Input: part model. Units: mm. Frame: model coordinates. A direction names the side the tool comes from. Round coordinates to 2 decimals unless told otherwise and drop trailing zeros. Loops run counter-clockwise (first coordinate to the right, second up) from the corner with the lowest first, then second, coordinate; pieces in that order, holes last.
(1) Cut plane C-C, the plane x = 0. Output: boundary loops of the cut face in (y, z) (1 decimal), and give its area (3 significant figures).
(2) Line query: line 1 (X direction, y = 328, z = 3); line 2 (X direction, y = 304.8, z = 1.85); line 3 (X direction, y = 330.2, z = 1.4). Output: solid intervals per line, ascending.
(3) Cut plane A-A, the plane x = -50.8. Output: boundary loops of the cut face in (y, z) (3 decimals).
(4) Draft query along Y for faces 3 (the face through (-12.7, 282, 2)), 4 (the face through (1.372, 281.552, 1.61)), 5 (the face through (-0.7, 246.15, 1.57)), 6 (the face through (-0.553, 327.708, 1.61)). Return one class per face: released by +Y, released by -Y, zero draft, split by the parting line, or undercut.
(5) Cut plane B-B, the plane z = 1.6. Output: boundary loops of the cut face in (x, y).
(6) Access query for faces 1 (the face through (-48, 317.5, 2)), 2 (the face through (-14, 316, 0)). Directions: +Z, -Z, +X, -X, +Y, -Y. A direction counts if a zero-diameter tool reaches every point of the face in a straight line with its end or side. Return the directions, or none.
(7) First-contact query: pin 1 Ø3 at (x, y) = (0, 254) entering from -Z; pin 2 Ø1.5 at (y, z) = (299.5, 1) entering from -X. Flat tips, straight axial feed; report the tip coordinate or a pass-through.
(8) Cut plane D-D, the plane y = 330.2. Output: boundary loops of the cut face in (x, z) (1 decimal).
from build123d import *

# Parameters (mm, degrees)
BOSS_EXTRUDE1_DEPTH        = 3.175
FILLET1_R                  = 6.35
F_10_CLEARANCE_HOLE1_D     = 5.1054
F_10_CLEARANCE_HOLE1_DEPTH = 9.906
F_10_CLEARANCE_HOLE1_TIP   = 1.533816902


with BuildPart() as part:
    # Sketch1 → Boss-Extrude1 (new body)
    with BuildSketch(Plane.XY):
        with BuildLine():
            Line((-12.7, 247.65), (-12.7, 317.5))
            Line((-12.7, 317.5), (-82.55, 317.5))
            Line((-82.55, 317.5), (-84.832797429, 335.762379435))
            ThreePointArc((-84.832797429, 335.762379435), (-83.292289329, 340.752446277), (-78.531832912, 342.9))
            Line((-78.531832912, 342.9), (6.35, 342.9))
            ThreePointArc((6.35, 342.9), (10.840128061, 341.040128061), (12.7, 336.55))
            Line((12.7, 336.55), (12.7, 251.668167088))
            ThreePointArc((12.7, 251.668167088), (10.552446277, 246.907710671), (5.562379435, 245.367202571))
            Line((5.562379435, 245.367202571), (-12.7, 247.65))
        make_face()
    extrude(amount=BOSS_EXTRUDE1_DEPTH)

    # Fillet1
    fillet1_edges = [part.edges().sort_by_distance(p)[0] for p in [
        (-12.7, 247.65, 1.5875),
        (-12.7, 317.5, 1.5875),
        (-82.55, 317.5, 1.5875),
    ]]
    fillet(fillet1_edges, radius=FILLET1_R)

    # #10 Clearance Hole1
    with Locations(Plane(origin=(0, 0, 0), x_dir=(-1, 0, 0), z_dir=(0, 0, -1))):
        with Locations((0, 330.2), (0, 304.8), (0, 279.4), (25.4, 330.2), (0, 254), (50.8, 330.2), (76.2, 330.2)):
            Hole(F_10_CLEARANCE_HOLE1_D / 2, depth=F_10_CLEARANCE_HOLE1_DEPTH)
            with Locations((0, 0, -(F_10_CLEARANCE_HOLE1_DEPTH + F_10_CLEARANCE_HOLE1_TIP / 2))):  # 118° drill point
                Cone(0, F_10_CLEARANCE_HOLE1_D / 2, F_10_CLEARANCE_HOLE1_TIP, mode=Mode.SUBTRACT)


solid = part.part
Reported:
1. outline: (246.1, 0) - (251.4, 0) - (251.4, 3.2) - (246.1, 3.2) - close; (256.6, 0) - (276.8, 0) - (276.8, 3.2) - (256.6, 3.2) - close; (282, 0) - (302.2, 0) - (302.2, 3.2) - (282, 3.2) - close; (307.4, 0) - (327.6, 0) - (327.6, 3.2) - (307.4, 3.2) - close; (332.8, 0) - (342.9, 0) - (342.9, 3.2) - (332.8, 3.2) - close
1. area: 243 mm2
2. line 1: x = -83.86 to -77.49, -74.91 to -52.09, -49.51 to -26.69, -24.11 to -1.29, 1.29 to 12.7
2. line 2: x = -12.7 to -2.55, 2.55 to 12.7
2. line 3: x = -84.14 to -78.75, -73.65 to -53.35, -48.25 to -27.95, -22.85 to -2.55, 2.55 to 12.7
3. outline: (317.5, 0) - (327.647, 0) - (327.647, 3.175) - (317.5, 3.175) - close; (332.753, 0) - (342.9, 0) - (342.9, 3.175) - (332.753, 3.175) - close
4. face 3: zero draft
4. face 4: undercut
4. face 5: released by -Y
4. face 6: undercut
5. outline: (-84.83, 335.76) - (-83.25, 323.06) arc R6.35 ccw to (-76.94, 317.5) - (-19.05, 317.5) arc R6.35 cw to (-12.7, 311.15) - (-12.7, 253.26) arc R6.35 ccw to (-7.14, 246.95) - (5.56, 245.37) arc R6.35 ccw to (12.7, 251.67) - (12.7, 336.55) arc R6.35 ccw to (6.35, 342.9) - (-78.53, 342.9) arc R6.35 ccw to start; hole circle Ø5.11 at (-76.2, 330.2); hole circle Ø5.11 at (-50.8, 330.2); hole circle Ø5.11 at (-25.4, 330.2); hole circle Ø5.11 at (0, 254); hole circle Ø5.11 at (0, 279.4); hole circle Ø5.11 at (0, 304.8); hole circle Ø5.11 at (0, 330.2)
6. face 1: +Z, -Z, -X, -Y
6. face 2: -Z, +X, -X, +Y, -Y
7. pin 1: passes through
7. pin 2: stops at x = -12.7
8. outline: (-84.1, 0) - (-78.8, 0) - (-78.8, 3.2) - (-84.1, 3.2) - close; (-73.6, 0) - (-53.4, 0) - (-53.4, 3.2) - (-73.6, 3.2) - close; (-48.2, 0) - (-28, 0) - (-28, 3.2) - (-48.2, 3.2) - close; (-22.8, 0) - (-2.6, 0) - (-2.6, 3.2) - (-22.8, 3.2) - close; (2.6, 0) - (12.7, 0) - (12.7, 3.2) - (2.6, 3.2) - close
